```python
from build123d import *

# Parameters (mm, degrees)
MODEL_R    = 1.75
MODEL_R_2  = 2.55
BASE_DEPTH = 6


with BuildPart() as part:
    # Model → Base (new body)
    with BuildSketch(Plane.XY):
        with BuildLine():
            Line((46.75, 74.75), (46.75, 6.25))
            ThreePointArc((46.75, 6.25), (44.919417382, 1.830582618), (40.5, 0))
            Line((40.5, 0), (-40.5, 0))
            ThreePointArc((-40.5, 0), (-44.919417382, 1.830582618), (-46.75, 6.25))
            Line((-46.75, 6.25), (-46.75, 74.75))
            ThreePointArc((-46.75, 74.75), (-44.919417382, 79.169417382), (-40.5, 81))
            Line((-40.5, 81), (40.5, 81))
            ThreePointArc((40.5, 81), (44.919417382, 79.169417382), (46.75, 74.75))
        make_face()
        with Locations((0, 4.5)):
            Circle(MODEL_R, mode=Mode.SUBTRACT)
        with Locations((8, 4.5)):
            Circle(MODEL_R, mode=Mode.SUBTRACT)
        with Locations((38.3, 50.35)):
            Circle(MODEL_R_2, mode=Mode.SUBTRACT)
        with Locations((38.3, 30.35)):
            Circle(MODEL_R_2, mode=Mode.SUBTRACT)
        with Locations((-38.3, 30.35)):
            Circle(MODEL_R_2, mode=Mode.SUBTRACT)
        with Locations((-38.3, 50.35)):
            Circle(MODEL_R_2, mode=Mode.SUBTRACT)
        with Locations((-8, 4.5)):
            Circle(MODEL_R, mode=Mode.SUBTRACT)
        with Locations((0, 54.4)):
            Circle(MODEL_R, mode=Mode.SUBTRACT)
        with Locations((26.5, 54.4)):
            Circle(MODEL_R, mode=Mode.SUBTRACT)
        with Locations((22, 40.4)):
            Circle(MODEL_R, mode=Mode.SUBTRACT)
        with Locations((-22, 40.4)):
            Circle(MODEL_R, mode=Mode.SUBTRACT)
        with Locations((-26.5, 54.4)):
            Circle(MODEL_R, mode=Mode.SUBTRACT)
        with BuildLine():
            Line((-3.1, 75.8), (-3.1, 72.6))
            ThreePointArc((-3.1, 72.6), (-5, 70.7), (-6.9, 72.6))
            Line((-6.9, 72.6), (-6.9, 75.8))
            ThreePointArc((-6.9, 75.8), (-5, 77.7), (-3.1, 75.8))
        make_face(mode=Mode.SUBTRACT)
        with BuildLine():
            Line((-9.75, 50.9), (-9.75, 44.4))
            ThreePointArc((-9.75, 44.4), (-8, 42.65), (-6.25, 44.4))
            Line((-6.25, 44.4), (-6.25, 50.9))
            ThreePointArc((-6.25, 50.9), (-8, 52.65), (-9.75, 50.9))
        make_face(mode=Mode.SUBTRACT)
        with BuildLine():
            Line((3.1, 72.6), (3.1, 75.8))
            ThreePointArc((3.1, 75.8), (5, 77.7), (6.9, 75.8))
            Line((6.9, 75.8), (6.9, 72.6))
            ThreePointArc((6.9, 72.6), (5, 70.7), (3.1, 72.6))
        make_face(mode=Mode.SUBTRACT)
        with BuildLine():
            Line((8.25, 17.25), (-8.25, 17.25))
            ThreePointArc((-8.25, 17.25), (-10, 15.5), (-8.25, 13.75))
            Line((-8.25, 13.75), (8.25, 13.75))
            ThreePointArc((8.25, 13.75), (10, 15.5), (8.25, 17.25))
        make_face(mode=Mode.SUBTRACT)
        with BuildLine():
            Line((9.75, 44.4), (9.75, 50.9))
            ThreePointArc((9.75, 50.9), (8, 52.65), (6.25, 50.9))
            Line((6.25, 50.9), (6.25, 44.4))
            ThreePointArc((6.25, 44.4), (8, 42.65), (9.75, 44.4))
        make_face(mode=Mode.SUBTRACT)
        with BuildLine():
            Line((-1.75, 29.85), (-1.75, 27.25))
            Line((-1.75, 27.25), (-12, 27.25))
            ThreePointArc((-12, 27.25), (-13.75, 25.5), (-12, 23.75))
            Line((-12, 23.75), (12, 23.75))
            ThreePointArc((12, 23.75), (13.75, 25.5), (12, 27.25))
            Line((12, 27.25), (1.75, 27.25))
            Line((1.75, 27.25), (1.75, 29.85))
            ThreePointArc((1.75, 29.85), (0, 31.6), (-1.75, 29.85))
        make_face(mode=Mode.SUBTRACT)
    extrude(amount=BASE_DEPTH)


solid = part.part
```
Geometry check sheet. Reference: the model listing, model coordinates, mm. A direction names the side the tool comes from. Coordinates: 2 decimals unless noted, no trailing zeros. Order: outer loops, then holes, each group sorted by start corner. A loop starts at its lowest first (then second) coordinate and runs counter-clockwise, first axis right, second up.
Item 1: Section check D-D (z = 2.9). Count the separate pieces of the cut face and the enclosed holes in it, plus the area to 3 significant figures.
Item 2: Section check B-B (x = -38.3). Enter the section's corners in (y, z).
Item 3: Scan lines: line 1 along Y through (x, z) = (38.3, 1.7); line 2 along Y through (x, z) = (-8, 2); line 3 along Y through (x, z) = (-22, 3.25). Record each from-to range of solid material in increasing order.
Item 4: Section check C-C (x = 5). Enter the section's corners in (y, z), plus the area to 3 significant figures.
Item 5: Mould release check, pull along Y, two halves, no side actions. Record for faces 3 (the cylindrical face through (5, 70.7, 3)), 4 (the flat face through (1, 41, 6)), 5 (the flat face through (-1, 81, 3)): released by +Y, released by -Y, zero draft, split by the parting line, or undercut.
Item 6: Tool access check on faces 1 (the flat face through (1, 41, 0)), 2 (the cylindrical face through (8.04, 52.65, 2.96)). Record the directions out of +Z, -Z, +X, -X, +Y, -Y that give a thin tool (end or side, any length) a straight path to the whole face; none if there is none.
Item 7: Section check A-A (y = 54.4). Enter the section's corners in (x, z).
Check sheet entries:
1. separate pieces: 1
1. enclosed holes: 18
1. area: 7,090 mm2
2. outline: (0, 0) - (27.8, 0) - (27.8, 6) - (0, 6) - close; (32.9, 0) - (47.8, 0) - (47.8, 6) - (32.9, 6) - close; (52.9, 0) - (81, 0) - (81, 6) - (52.9, 6) - close
3. line 1: y = 0 to 27.8, 32.9 to 47.8, 52.9 to 81
3. line 2: y = 0 to 2.75, 6.25 to 13.75, 17.25 to 23.75, 27.25 to 42.65, 52.65 to 81
3. line 3: y = 0 to 38.65, 42.15 to 81
4. outline: (0, 0) - (13.75, 0) - (13.75, 6) - (0, 6) - close; (17.25, 0) - (23.75, 0) - (23.75, 6) - (17.25, 6) - close; (27.25, 0) - (70.7, 0) - (70.7, 6) - (27.25, 6) - close; (77.7, 0) - (81, 0) - (81, 6) - (77.7, 6) - close
4. area: 402 mm2
5. face 3: undercut
5. face 4: zero draft
5. face 5: released by +Y
6. face 1: -Z, +X, -X, +Y, -Y
6. face 2: +Z, -Z
7. outline: (-46.75, 0) - (-28.25, 0) - (-28.25, 6) - (-46.75, 6) - close; (-24.75, 0) - (-1.75, 0) - (-1.75, 6) - (-24.75, 6) - close; (1.75, 0) - (24.75, 0) - (24.75, 6) - (1.75, 6) - close; (28.25, 0) - (46.75, 0) - (46.75, 6) - (28.25, 6) - close
